Work out the finished part from the listing and answer in its coordinate system (mm). Round coordinates to 2 decimals unless told otherwise and drop trailing zeros. Order: outer loops, then holes, each group sorted by start corner. A loop starts at its lowest first (then second) coordinate and runs counter-clockwise, first axis right, second up. Notation, with made-up numbers: (58, 36.5) -> (109, 36.5) arc R19 cw to (109, 72.5) -> close; hole circle Ø4 at (14.25, 20). An arc over 180 degrees is marked (long way). Use a Markdown table: item, result. Add a question column.
Item 1: A cutting plane is placed at B-B, the plane x = 0. Determine the outline of the cut face in (y, z).
Item 2: A cutting plane is placed at C-C, the plane x = -24. Determine the outline of the cut face in (y, z), plus the area to 3 significant figures.
Item 3: Flat-ended cylindrical pins translate along their axes: P1, Ø2, axis at y = -16.5, z = 1.5, coming from the +X side; P2, Ø1, axis at y = -6.5, z = 7, coming from the -X side; P3, Ø2.5, axis at x = -24, y = 36, coming from the -Z side; P4, Ø1, axis at y = -31, z = 8.5, coming from the +X side. Find the tip coordinate at first contact, or state that the pin passes through.
Item 4: A cutting plane is placed at D-D, the plane y = -28.4. Determine the outline of the cut face in (x, z).
Item 5: A cutting plane is placed at A-A, the plane y = 36. Determine the outline of the cut face in (x, z).
Item 6: Find the intervals of material crossed by L1, parallel to Y at x = 24, z = 7.5; L2, parallel to Y at x = -23, z = 8.5; L3, parallel to Y at x = 0, z = 6, in increasing order. Write a range as [from, to].
from build123d import *

# Parameters (mm, degrees)
F1_DEPTH = 10
F3_D     = 5
F4_D     = 3


with BuildPart() as f1:
    # F0 (on Top) → F1 (new body)
    with BuildSketch(Plane.XY):
        Polygon((35, -5), (35, 55), (-35, 55), (-35, -5), (-30, -55), (30, -55), align=None)
    extrude(amount=F1_DEPTH)

    # F3 (through all)
    with Locations(Plane.XY.offset(10)):
        with Locations((0, -28.4)):
            Hole(F3_D / 2)

    # F4 (through all)
    with Locations(Plane.XY.offset(10)):
        with Locations((-24, 36), (24, 36), (24, -46), (-24, -46)):
            Hole(F4_D / 2)


solid = f1.part
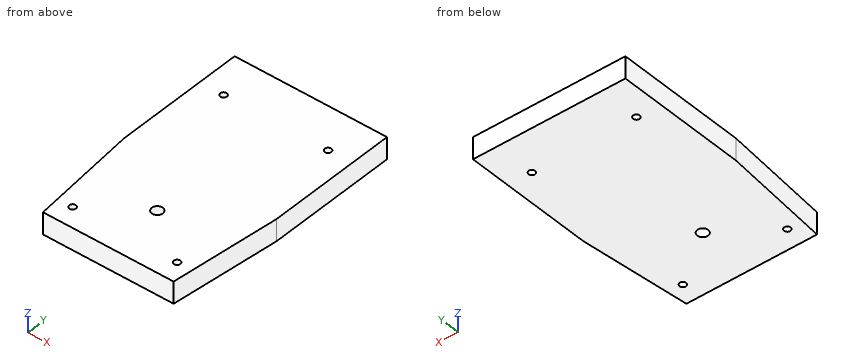
Reported:
| question | item | result |
|---|---|---|
| 1 | outline | (-55, 0) -> (-30.9, 0) -> (-30.9, 10) -> (-55, 10) -> close; (-25.9, 0) -> (55, 0) -> (55, 10) -> (-25.9, 10) -> close |
| 2 | outline | (-55, 0) -> (-47.5, 0) -> (-47.5, 10) -> (-55, 10) -> close; (-44.5, 0) -> (34.5, 0) -> (34.5, 10) -> (-44.5, 10) -> close; (37.5, 0) -> (55, 0) -> (55, 10) -> (37.5, 10) -> close |
| 2 | area | 1,040 mm² |
| 3 | P1 | x = 33.95 |
| 3 | P2 | x = -34.9 |
| 3 | P3 | through |
| 3 | P4 | x = 32.45 |
| 4 | outline | (-32.66, 0) -> (-2.5, 0) -> (-2.5, 10) -> (-32.66, 10) -> close; (2.5, 0) -> (32.66, 0) -> (32.66, 10) -> (2.5, 10) -> close |
| 5 | outline | (-35, 0) -> (-25.5, 0) -> (-25.5, 10) -> (-35, 10) -> close; (-22.5, 0) -> (22.5, 0) -> (22.5, 10) -> (-22.5, 10) -> close; (25.5, 0) -> (35, 0) -> (35, 10) -> (25.5, 10) -> close |
| 6 | L1 | [-55, -47.5], [-44.5, 34.5], [37.5, 55] |
| 6 | L2 | [-55, -47.12], [-44.88, 34.88], [37.12, 55] |
| 6 | L3 | [-55, -30.9], [-25.9, 55] |
